Autodesk Fusion 360 part; units mm, degrees
sketch "Sketch1" plane through (0, 0, 0) normal (1, 0, 0) x (0, 0, -1)
  line L0 (0, 0) -> (-150, 0)
  line L1 (-150, 0) -> (-150, 25)
  line L2 (-150, 25) -> (0, 25)
  line L3 (0, 25) -> (0, 0)
  line L4 (-10, 0) -> (-140, 0)
  line L5 (-140, 0) -> (-140, 25)
  line L6 (-140, 25) -> (-10, 25)
  line L7 (-10, 25) -> (-10, 0)
  line L8 (-140, 20) -> (-150, 20)
  line L9 (-150, 20) -> (-150, 5)
  line L10 (-150, 5) -> (-140, 5)
  line L11 (-140, 5) -> (-140, 20)
  line L12 (-10, 5) -> (0, 5)
  line L13 (0, 5) -> (0, 20)
  line L14 (0, 20) -> (-10, 20)
  line L15 (-10, 20) -> (-10, 5)
  dimension "d1" = 150
  dimension "d2" = 25
  dimension "d3" = 130
  dimension "d4" = 25
extrude "Extrude1" add sketch "Sketch1" along normal blind 10 contours L0 L2 L4 L5 L6 L7 L11 L15 | L3 L7 L12 L13 L14 L15 | L1 L5 L8 L9 L10 L11
sketch "Sketch2" plane through (0, 0, 0) normal (0, -1, 0) x (1, 0, 0)
  line L0 (0, 140) -> (0, 10)
  line L1 (0, 10) -> (10, 10)
  line L2 (10, 10) -> (10, 140)
  line L3 (10, 140) -> (0, 140)
  line L4 (0, 140) -> (10, 140)
  line L5 (10, 140) -> (10, 88)
  line L6 (10, 88) -> (0, 88)
  line L7 (0, 88) -> (0, 140)
  line L8 (0, 10) -> (10, 10)
  line L9 (10, 10) -> (10, 62)
  line L10 (10, 62) -> (0, 62)
  line L11 (0, 62) -> (0, 10)
  line L12 (0, 140) -> (10, 140)
  line L13 (10, 140) -> (10, 138)
  line L14 (10, 138) -> (0, 138)
  line L15 (0, 138) -> (0, 140)
  line L16 (0, 10) -> (10, 10)
  line L17 (10, 10) -> (10, 12)
  line L18 (10, 12) -> (0, 12)
  line L19 (0, 12) -> (0, 10)
  dimension "d7" = 52
  dimension "d8" = 52
  dimension "d9" = 2
extrude "Extrude2" cut sketch "Sketch2" against normal blind 20 contours L0 L2 L5 L6 L7 L14 | L0 L2 L9 L10 L11 L18
fillet "Fillet1" radius 5 4 edges at (5, 20, 138) (5, 20, 88) (5, 20, 62) (5, 20, 12)
The listing builds one solid part. Answer for the finished solid, in the listing's coordinates (mm). A direction names the side the tool comes from. Coordinates: 2 decimals unless noted, no trailing zeros. Loops run counter-clockwise (first coordinate to the right, second up) from the corner with the lowest first, then second, coordinate; pieces in that order, holes last. Notation, with made-up numbers: (87, -32) - (131, -32) arc R17 ccw to (131, -11) - close; hole circle Ø4 at (64.25, 47). An arc over 180 degrees is marked (long way). Use a Markdown table: item, result. Add a question column.
1) Given pin 1 (1.5 mm diameter, centred on x = 9, y = 3.5, fed in from +Z); pin 2 (5 mm diameter, centred on x = 3.5, z = 6, fed in from +Y); pin 3 (4 mm diameter, centred on x = 6, y = 23, fed in from -Z), each flat-ended and moving along its own axis, determine where each tip first touches the part or whether it passes through.
2) Find the intervals of material crossed by line 1 (Z direction, x = 1.5, y = 11.5); line 2 (Z direction, x = 6, y = 3); line 3 (Y direction, x = 4.5, z = 34.5), in increasing order.
3) The part is cut by section D-D, the plane z = 120. Give the vertices of the cut face in (x, y).
4) The part is cut by section B-B, the plane x = 4. Give the vertices of the cut face in (y, z), and give its area (3 significant figures).
5) The part is cut by section A-A, the plane y = 12.5. Give the vertices of the cut face in (x, z).
6) The mould has two halves that part along Z. Classify faces 1 (the flat face through (5, 13, 0)), 2 (the flat face through (5, 20, 37)), 3 (the flat face through (5, 0, 75)): released by +Z, released by -Z, zero draft, split by the parting line, or undercut.
7) The part is cut by section C-C, the plane y = 2.5. Give the vertices of the cut face in (x, z).
8) For faces 4 (the flat face through (5, 23, 10)), 5 (the flat face through (5, 12, 150)), 6 (the flat face through (5, 20, 145)), 7 (the flat face through (5, 20, 113)), 8 (the flat face through (5, 5, 5)), determine the directions among +Z, -Z, +X, -X, +Y, -Y from which every point of the face is accessible in a straight line to the end or side of a thin tool.
Here are the results:
| question | item | result |
|---|---|---|
| 1 | pin 1 | stops at z = 140 |
| 1 | pin 2 | stops at y = 20 |
| 1 | pin 3 | stops at z = 10 |
| 2 | line 1 | z = 0 to 12, 62 to 88, 138 to 150 |
| 2 | line 2 | z = 10 to 12, 62 to 88, 138 to 140 |
| 2 | line 3 | y = 20 to 25 |
| 3 | outline | (0, 20) - (10, 20) - (10, 25) - (0, 25) - close |
| 4 | outline | (0, 10) - (5, 10) - (5, 0) - (20, 0) - (20, 10) - (25, 10) - (25, 140) - (20, 140) - (20, 150) - (5, 150) - (5, 140) - (0, 140) - (0, 138) - (15, 138) arc R5 cw to (20, 133) - (20, 93) arc R5 cw to (15, 88) - (0, 88) - (0, 62) - (15, 62) arc R5 cw to (20, 57) - (20, 17) arc R5 cw to (15, 12) - (0, 12) - close |
| 4 | area | 1,570 mm^2 |
| 5 | outline | (0, 0) - (10, 0) - (10, 12) - (0, 12) - close; (0, 62) - (10, 62) - (10, 88) - (0, 88) - close; (0, 138) - (10, 138) - (10, 150) - (0, 150) - close |
| 6 | face 1 | released by -Z |
| 6 | face 2 | undercut |
| 6 | face 3 | zero draft |
| 7 | outline | (0, 10) - (10, 10) - (10, 12) - (0, 12) - close; (0, 62) - (10, 62) - (10, 88) - (0, 88) - close; (0, 138) - (10, 138) - (10, 140) - (0, 140) - close |
| 8 | face 4 | -Z, +X, -X, +Y |
| 8 | face 5 | +Z, +X, -X, +Y, -Y |
| 8 | face 6 | +Z, +X, -X, +Y |
| 8 | face 7 | +X, -X, -Y |
| 8 | face 8 | -Z, +X, -X, -Y |
